Geometry: final body of the model. Coordinates: model frame, mm. A direction names the side the tool comes from. Give positions to 0.01 mm unless a question says otherwise; leave off trailing zeros. Loops run counter-clockwise (first coordinate to the right, second up) from the corner with the lowest first, then second, coordinate; pieces in that order, holes last. Notation, with made-up numbers: M -38.75,-26 L -19.75,-26 A23 cw -19.75,2 Z; hole C -6.5,6 d9. An arc over 180 degrees is marked long. Put each result on its own line as item: value.
Autodesk Fusion 360 part; units mm, degrees
sketch "Sketch1" plane through (0, 0, 0) normal (0, 0, 1) x (1, 0, 0)
  line L0 (5, 0) -> (120, 0)
  line L1 (125, 5) -> (125, 120)
  line L2 (120, 125) -> (5, 125)
  line L3 (0, 120) -> (0, 5)
  arc A0 (125, 120) -> (120, 125) centre (120, 120) ccw
  arc A1 (5, 125) -> (0, 120) centre (5, 120) ccw
  arc A2 (0, 5) -> (5, 0) centre (5, 5) ccw
  arc A3 (120, 0) -> (125, 5) centre (120, 5) ccw
  circle A4 centre (12, 32.5) radius 2.5
  circle A5 centre (113, 32.5) radius 2.5
  circle A6 centre (12, 92.5) radius 2.5
  line L4 (45, 80) -> (80, 80)
  line L5 (80, 80) -> (80, 45)
  line L6 (80, 45) -> (45, 45)
  line L7 (45, 45) -> (45, 80)
  dimension "d3" = 10
  dimension "d4" = 10
  dimension "d5" = 10
  dimension "d6" = 10
  dimension "d7" = 5
  dimension "d8" = 12
  dimension "d9" = 32.5
  dimension "d10" = 5
  dimension "d11" = 12
  dimension "d12" = 32.5
  dimension "d13" = 5
  dimension "d15" = 12
  dimension "d16" = 32.5
  dimension "d81" = 35
  dimension "d82" = 35
  dimension "d83" = 45
  dimension "d84" = 45
  dimension "d85" = 45
  dimension "d86" = 45
extrude "Extrude1" add sketch "Sketch1" along normal blind 5
sketch "Sketch2" plane through (0, 0, 5) normal (0, 0, 1) x (-1, 0, 0)
  circle A0 centre (-12, -72.5) radius 3
  line L0 (0, -120) -> (0, -5)
  circle A1 centre (-12, -52.5) radius 3
  circle A2 centre (-113, -52.5) radius 3
  line L1 (-125, -5) -> (-125, -120)
  circle A3 centre (-113, -72.5) radius 3
  circle A4 centre (-113, -92.5) radius 2.5
  line L2 (-120, -125) -> (-5, -125)
  point P0 (-12, -92.5)
  point P1 (-12, -32.5)
  point P2 (-113, -32.5)
  dimension "d65" = 6
  dimension "d66" = 20
  dimension "d67" = 12
  dimension "d68" = 6
  dimension "d69" = 20
  dimension "d70" = 12
  dimension "d71" = 20
  dimension "d72" = 6
  dimension "d73" = 12
  dimension "d74" = 6
  dimension "d75" = 12
  dimension "d148" = 5
  dimension "d149" = 20
  dimension "d150" = 20
  dimension "d151" = 20
  dimension "d152" = 32.5
  dimension "d153" = 12
sketch "Sketch3" plane through (0, 0, 5) normal (0, 0, 1) x (-1, 0, 0)
extrude "Extrude2" add sketch "Sketch2" against normal blind 5 contours A0 | A1 | A2 | A3
extrude "Extrude3" cut sketch "Sketch2" against normal blind 5 contours A0 | A1 | A2 | A3
sketch "Sketch4" plane through (0, 0, 5) normal (0, 0, 1) x (-1, 0, 0)
  circle A0 centre (-113, -92.5) radius 2.5
  line L0 (-120, -125) -> (-5, -125)
  line L1 (-125, -5) -> (-125, -120)
  dimension "d145" = 5
  dimension "d146" = 32.5
  dimension "d147" = 12
extrude "Extrude4" cut sketch "Sketch4" against normal blind 5
Item 1: Section D-D on z = 3.55. Count the separate pieces of the cut face and the enclosed holes in it, then the cut area to 3 significant figures.
Output values:
separate pieces: 1
enclosed holes: 9
area: 14,200 mm²
Item 2: Section B-B on y = 78. Output: boundary loops of the cut face in (x, z), then the cut area to 3 significant figures.
Output values:
outline: M 0,0 L 45,0 L 45,5 L 0,5 Z; M 80,0 L 125,0 L 125,5 L 80,5 Z
area: 450 mm²
Item 3: Line query: probe 1 along Y at (x, z) = (113, 2.5); probe 2 along X at (y, z) = (72.5, 1.7); probe 3 along Y at (x, z) = (73, 4.35). Output: solid intervals per line, ascending. Write a range as [from, to].
Output values:
probe 1: [0, 30], [35, 49.5], [55.5, 69.5], [75.5, 90], [95, 125]
probe 2: [0, 9], [15, 45], [80, 110], [116, 125]
probe 3: [0, 45], [80, 125]
Item 4: Section C-C on x = 113. Output: boundary loops of the cut face in (y, z), then the cut area to 3 significant figures.
Output values:
outline: M 0,0 L 30,0 L 30,5 L 0,5 Z; M 35,0 L 49.5,0 L 49.5,5 L 35,5 Z; M 55.5,0 L 69.5,0 L 69.5,5 L 55.5,5 Z; M 75.5,0 L 90,0 L 90,5 L 75.5,5 Z; M 95,0 L 125,0 L 125,5 L 95,5 Z
area: 515 mm²
Item 5: Mould query, pull axis X, two halves, no side actions, for faces 3 (the flat face through (63, 125, 2)), 4 (the cylindrical face through (1, 123, 2)), 5 (the cylindrical face through (12.65, 75.43, 2.54)). Classes: pulls with the +X half, pulls with the -X half, needs draft (parallel to the pull), parting line crosses it, or undercut.
Output values:
face 3: needs draft
face 4: pulls with the -X half
face 5: undercut
Item 6: Set-up query: faces 1 (the flat face through (62, 80, 2)), 2 (the cylindrical face through (2, 1, 2)). Return all of +Z, -Z, +X, -X, +Y, -Y with unobstructed straight access to the full face (end or side cutting, diameter ignored); none if empty.
Output values:
face 1: +Z, -Z
face 2: +Z, -Z, -X, -Y
Item 7: Pin query (flat end, axial travel): pin 1 Ø5 at (x, y) = (113, 52.5) entering from +Z. Return the tip coordinate at first contact, or that it passes through.
Output values:
pin 1: through
Item 8: Section A-A on y = 92.5. Output: boundary loops of the cut face in (x, z).
Output values:
outline: M 0,0 L 9.5,0 L 9.5,5 L 0,5 Z; M 14.5,0 L 110.5,0 L 110.5,5 L 14.5,5 Z; M 115.5,0 L 125,0 L 125,5 L 115.5,5 Z
